Could you check a few things on this model? Use its own coordinates, in mm. Face numbers are marked on the shaded views. A direction names the side the tool comes from. Give positions to 0.01 mm unless a question says otherwise; leave off trailing zeros. Order: outer loops, then holes, each group sorted by start corner. A loop starts at its lowest first (then second) coordinate and runs counter-clockwise, first axis right, second up. Notation, with made-up numbers: M 64,38.5 L 98,38.5 A21 cw 98,52.5 Z; hole C 77.5,88 d4. An arc over 180 degrees is marked long. Return JSON: item names as keys, results as strings. Group by question number.
```python
from build123d import *

# Parameters (mm, degrees)
SKETCH1_W           = 66
SKETCH1_H           = 40
SKETCH1_R           = 2.5
BOSS_EXTRUDE1_DEPTH = 3
BOSS_EXTRUDE2_DEPTH = 65
SKETCH3_W           = 6
SKETCH3_H           = 4
BOSS_EXTRUDE3_DEPTH = 32


with BuildPart() as part:
    # Sketch1 → Boss-Extrude1 (new body)
    with BuildSketch(Plane(origin=(0, 0, 0), x_dir=(1, 0, 0), z_dir=(0, 1, 0))):
        with Locations((-78.704067838, 45.994872636)):
            Rectangle(SKETCH1_W, SKETCH1_H)
        with Locations(Location((-105.204067838, 59.494872636, 0), (0, 0, 270))):
            Circle(SKETCH1_R, mode=Mode.SUBTRACT)
        with Locations(Location((-105.204067838, 32.494872636, 0), (0, 0, 270))):
            Circle(SKETCH1_R, mode=Mode.SUBTRACT)
        with Locations(Location((-52.204067838, 59.494872636, 0), (0, 0, 270))):
            Circle(SKETCH1_R, mode=Mode.SUBTRACT)
        with Locations(Location((-52.204067838, 32.494872636, 0), (0, 0, 270))):
            Circle(SKETCH1_R, mode=Mode.SUBTRACT)
    extrude(amount=BOSS_EXTRUDE1_DEPTH)

    # Sketch2 → Boss-Extrude2 (add)
    with BuildSketch(Plane(origin=(0, 3, 0), x_dir=(1, 0, 0), z_dir=(0, 1, 0))):
        Polygon((-98.704067838, 65.994872636), (-58.704067838, 65.994872636), (-58.704067838, 25.994872636), (-71.704067838, 25.994872636), (-71.704067838, 29.994872636), (-62.704067838, 29.994872636), (-62.704067838, 61.994872636), (-94.704067838, 61.994872636), (-94.704067838, 29.994872636), (-85.704067838, 29.994872636), (-85.704067838, 25.994872636), (-98.704067838, 25.994872636), align=None)
    extrude(amount=BOSS_EXTRUDE2_DEPTH)

    # Sketch3 → Boss-Extrude3 (add)
    with BuildSketch(Plane.XY.offset(-61.994872636)):
        with Locations((-91.704067838, 33)):
            Rectangle(SKETCH3_W, SKETCH3_H)
        with Locations((-65.704067838, 33)):
            Rectangle(SKETCH3_W, SKETCH3_H)
    extrude(amount=BOSS_EXTRUDE3_DEPTH)


solid = part.part
```
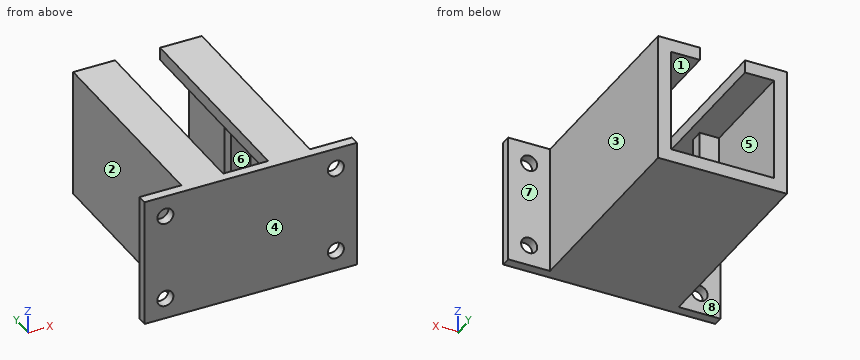
1. I need wall thicknesses on L1, parallel to X at y = 9.5, z = -41; L2, parallel to Y at x = -65, z = -59; L3, parallel to Z at x = -86, y = 65.5. Which ranges of each line are inside material? Lowest first, please. Write a range as from..to.
2. For pin 1 (3 mm diameter, centred on x = -91.5, z = -42, fed in from +Y); pin 2 (1.2 mm diameter, centred on y = 32, z = -28, fed in from +X); pin 3 (1 mm diameter, centred on y = 52.5, z = -51, fed in from -X), each with a flat end and sliding along its axis, tell me the tip position at first contact or that it passes through.
3. Imagine slicing it at D-D, the plane z = -56. Please give me the cut outline in (x, y).
4. Imagine slicing it at A-A, the plane z = -32.5. Please give me the cut outline in (x, y).
5. Which directions (+Z, -Z, +X, -X, +Y, -Y) give clear straight access to the entire face, cutting with the end or side of a thin tool? Please do the marked faces 5, 6, 7 and 8.
6. Imagine slicing it at B-B, the plane x = -104. Please give me the cut outline in (y, z).
7. If we mould it in two halves opening along X, with no side actions, what happens to the marked faces 1, 2, 3 and 4? For each: pulls with the +X half, pulls with the -X half, needs draft (parallel to the pull), parting line crosses it, or undercut.
8. Imagine slicing it at C-C, the plane y = 38.5. Please give me the cut outline in (x, z).
Values:
{
 "1": {"L1": "x = -98.7..-94.7, -62.7..-58.7", "L2": "y = 0..3, 31..35", "L3": "z = -65.99..-61.99, -29.99..-25.99"},
 "2": {"pin 1": "stops at y = 35", "pin 2": "stops at x = -58.7", "pin 3": "stops at x = -98.7"},
 "3": {"outline": "M -111.7,0 L -45.7,0 L -45.7,3 L -58.7,3 L -58.7,68 L -62.7,68 L -62.7,35 L -68.7,35 L -68.7,31 L -62.7,31 L -62.7,3 L -94.7,3 L -94.7,31 L -88.7,31 L -88.7,35 L -94.7,35 L -94.7,68 L -98.7,68 L -98.7,3 L -111.7,3 Z"},
 "4": {"outline": "M -111.7,0 L -107.7,0 L -107.7,3 L -111.7,3 Z; M -102.7,0 L -54.7,0 L -54.7,3 L -58.7,3 L -58.7,68 L -62.7,68 L -62.7,35 L -68.7,35 L -68.7,31 L -62.7,31 L -62.7,3 L -94.7,3 L -94.7,31 L -88.7,31 L -88.7,35 L -94.7,35 L -94.7,68 L -98.7,68 L -98.7,3 L -102.7,3 Z; M -49.7,0 L -45.7,0 L -45.7,3 L -49.7,3 Z"},
 "5": {"face 5": "+Y", "face 6": "none", "face 7": "+Z, -Z, +X, +Y", "face 8": "+Z, -Z, -X, +Y"},
 "6": {"outline": "M 0,-65.99 L 3,-65.99 L 3,-61.69 L 0,-61.69 Z; M 0,-57.3 L 3,-57.3 L 3,-34.69 L 0,-34.69 Z; M 0,-30.3 L 3,-30.3 L 3,-25.99 L 0,-25.99 Z"},
 "7": {"face 1": "undercut", "face 2": "pulls with the -X half", "face 3": "pulls with the +X half", "face 4": "needs draft"},
 "8": {"outline": "M -98.7,-65.99 L -58.7,-65.99 L -58.7,-25.99 L -71.7,-25.99 L -71.7,-29.99 L -62.7,-29.99 L -62.7,-61.99 L -94.7,-61.99 L -94.7,-29.99 L -85.7,-29.99 L -85.7,-25.99 L -98.7,-25.99 Z"}
}
